```python
from build123d import *
from build123d.topology import SkipClean

# Parameters (mm, degrees)
SKETCH7_W       = 80
SKETCH7_H       = 28
EXTRUDE2_DEPTH  = 4
SKETCH8_W       = 28
SKETCH8_H       = 20
EXTRUDE3_DEPTH  = 9.5
EXTRUDE6_DEPTH  = 28
SKETCH15_R      = 7.5
EXTRUDE7_DEPTH  = 25
SKETCH16_W      = 3
SKETCH16_H      = 3
SKETCH8_4_W     = 28
SKETCH8_4_H     = 20
EXTRUDE8_DEPTH  = 9.5
EXTRUDE9_DEPTH  = 28
SKETCH19_R      = 7.5
EXTRUDE10_DEPTH = 25
SKETCH20_W      = 3
SKETCH20_H      = 3
FILLET1_R       = 2.5
EXTRUDE11_DEPTH = 16
SKETCH25_W      = 28
SKETCH25_H      = 5
EXTRUDE13_DEPTH = 12
EXTRUDE14_REACH = 90.69
FILLET11_R      = 2
SKETCH27_W      = 28
SKETCH27_H      = 5
EXTRUDE15_DEPTH = 12
EXTRUDE16_REACH = 90.69
FILLET14_R      = 2
SKETCH30_W      = 3
SKETCH30_H      = 3
EXTRUDE17_DEPTH = 12
SKETCH31_W      = 3
SKETCH31_H      = 3
EXTRUDE18_DEPTH = 12
SKETCH32_R      = 4
EXTRUDE19_DEPTH = 40
FILLET15_R      = 2
FILLET16_R      = 2
FILLET17_R      = 2
FILLET18_R      = 2
FILLET19_R      = 2
FILLET20_R      = 2
FILLET21_R      = 2
SKETCH33_R      = 1.5
EXTRUDE20_DEPTH = 59.523499692


with BuildPart() as part:
    # Sketch7 → Extrude2 (new body)
    with BuildSketch(Plane(origin=(0, 0, 0), x_dir=(1, 0, 0), z_dir=(0, 1, 0))):
        with Locations((0, 23)):
            Rectangle(SKETCH7_W, SKETCH7_H)
    extrude(amount=EXTRUDE2_DEPTH)


with BuildPart() as body_2:
    # Sketch8 → Extrude3 (new body)
    with BuildSketch(Plane(origin=(0, 4, 0), x_dir=(1, 0, 0), z_dir=(0, 1, 0))):
        with Locations((-23, 24)):
            Rectangle(SKETCH8_W, SKETCH8_H)
    extrude(amount=EXTRUDE3_DEPTH)

    # Sketch10 → Extrude6 (cut)
    with BuildSketch(Plane(origin=(-9, 0, 0), x_dir=(0, 0, -1), z_dir=(1, 0, 0))):
        with BuildLine():
            Line((31.5, 13.5), (24, 13.5))
            Line((24, 13.5), (16.5, 13.5))
            ThreePointArc((16.5, 13.5), (17.126403912, 10.499387259), (18.900980486, 8))
            Line((18.900980486, 8), (29.099019514, 8))
            ThreePointArc((29.099019514, 8), (30.873596088, 10.499387259), (31.5, 13.5))
        make_face()
    extrude(amount=-EXTRUDE6_DEPTH, mode=Mode.SUBTRACT)

    # Sketch15 → Extrude7 (cut)
    with SkipClean():  # the faces are left unmerged after this step: merging them gives an invalid solid
        with BuildSketch(Plane.ZY.offset(35.5)):
            with Locations((-24, 13.5)):
                Circle(SKETCH15_R)
        extrude(amount=-EXTRUDE7_DEPTH, mode=Mode.SUBTRACT)


with BuildPart() as cut_sweep1_tool:
    # Cut-Sweep1: sweep along a path in Sketch17
    with SkipClean():  # the faces are left unmerged after this step: merging them gives an invalid solid
        with BuildLine(Plane(origin=(-23, 0, 0), x_dir=(0, 0, -1), z_dir=(1, 0, 0))) as cut_sweep1_path:
            CenterArc((24, 13.5), 12.806248475, 0, 360)
        # Sketch16 → Cut-Sweep1 (sweep)
        with BuildSketch(Plane.XY.offset(-14)):
            with Locations((-23, 5.5)):
                Rectangle(SKETCH16_W, SKETCH16_H)
        sweep(path=cut_sweep1_path.line)


with BuildPart() as part_1:
    with SkipClean():  # the faces are left unmerged after this step: merging them gives an invalid solid
        add(part.part)

        # Cut-Sweep1: cut by cut_sweep1_tool
        add(cut_sweep1_tool.part, mode=Mode.SUBTRACT)

    # Sketch8<4> → Extrude8 (add)
    with BuildSketch(Plane(origin=(0, 4, 0), x_dir=(1, 0, 0), z_dir=(0, 1, 0))):
        with Locations((23, 24)):
            Rectangle(SKETCH8_4_W, SKETCH8_4_H)
    extrude(amount=EXTRUDE8_DEPTH)

    # Sketch18 → Extrude9 (cut)
    with BuildSketch(Plane(origin=(37, 0, 0), x_dir=(0, 0, -1), z_dir=(1, 0, 0))):
        with BuildLine():
            Line((18.900980486, 8), (29.099019514, 8))
            ThreePointArc((29.099019514, 8), (30.873596088, 10.499387259), (31.5, 13.5))
            Line((31.5, 13.5), (16.5, 13.5))
            ThreePointArc((16.5, 13.5), (17.126403912, 10.499387259), (18.900980486, 8))
        make_face()
    extrude(amount=-EXTRUDE9_DEPTH, mode=Mode.SUBTRACT)

    # Sketch19 → Extrude10 (cut)
    with BuildSketch(Plane(origin=(35.5, 0, 0), x_dir=(0, 0, -1), z_dir=(1, 0, 0))):
        with Locations((24, 13.5)):
            Circle(SKETCH19_R)
    extrude(amount=-EXTRUDE10_DEPTH, mode=Mode.SUBTRACT)

    # Cut-Sweep2: sweep along a path in Sketch21
    with BuildLine(Plane(origin=(23, 0, 0), x_dir=(0, 0, -1), z_dir=(1, 0, 0))) as cut_sweep2_path:
        CenterArc((24, 13.5), 12.806248475, 0, 360)
    # Sketch20 → Cut-Sweep2 (sweep, cut)
    with BuildSketch(Plane.XY.offset(-14)):
        with Locations((23, 5.5)):
            Rectangle(SKETCH20_W, SKETCH20_H)
    sweep(path=cut_sweep2_path.line, mode=Mode.SUBTRACT)

    # Fillet1
    fillet1_edges = [part_1.edges().sort_by_distance(p)[0] for p in [
        (-40, 2, -37),
        (40, 2, -37),
    ]]
    fillet(fillet1_edges, radius=FILLET1_R)

    # Sketch22 → Extrude11 (add)
    with BuildSketch(Plane(origin=(0, 0, 0), x_dir=(1, 0, 0), z_dir=(0, 1, 0))):
        Polygon((36.784969303, -11.093941854), (40, 9), (-40, 9), (-32, -41), (-16, -41), (-11.215030697, -11.093941854), align=None)
        Polygon((12.66820222, 4), (11.053171523, -6.093941854), (-5.351435136, -6.093941854), (-3.73640444, 4), align=None, mode=Mode.SUBTRACT)
        Polygon((17.73179778, 4), (34.13640444, 4), (32.521373743, -6.093941854), (16.116767084, -6.093941854), align=None, mode=Mode.SUBTRACT)
    extrude(amount=EXTRUDE11_DEPTH)



with BuildPart() as body_2_1:
    with SkipClean():  # the faces are left unmerged after this step: merging them gives an invalid solid
        add(body_2.part)

        # Cut-Sweep1: cut by cut_sweep1_tool
        add(cut_sweep1_tool.part, mode=Mode.SUBTRACT)


with BuildPart() as part_2:
    with SkipClean():  # the faces are left unmerged after this step: merging them gives an invalid solid
        add(part_1.part)

        add(body_2_1.part)  # Extrude13 merges body 2
        # Sketch25 → Extrude13 (add)
        with BuildSketch(Plane(origin=(0, 4, 0), x_dir=(-1, 0, 0), z_dir=(0, 1, 0))):
            with Locations((23, -11.5)):
                Rectangle(SKETCH25_W, SKETCH25_H)
        extrude(amount=EXTRUDE13_DEPTH)

    # Sketch26 → Extrude14 (cut, up to next)
    with BuildSketch(Plane.ZY.offset(37), mode=Mode.PRIVATE) as extrude14_sk1:
        Polygon((-14, 13.5), (-9, 16), (-14, 16), align=None)
    extrude14_tool1 = extrude(extrude14_sk1.sketch, amount=-EXTRUDE14_REACH, mode=Mode.PRIVATE) & part_2.part
    add(extrude14_tool1.solids().sort_by_distance((-37, 15.166667, -12.333333))[0], mode=Mode.SUBTRACT)

    # Fillet11
    fillet11_edges = [part_2.edges().sort_by_distance(p)[0] for p in [
        (-9, 10, -9),
    ]]
    fillet(fillet11_edges, radius=FILLET11_R)

    # Sketch27 → Extrude15 (add)
    with SkipClean():  # the faces are left unmerged after this step: merging them gives an invalid solid
        with BuildSketch(Plane(origin=(0, 4, 0), x_dir=(-1, 0, 0), z_dir=(0, 1, 0))):
            with Locations((-23, -11.5)):
                Rectangle(SKETCH27_W, SKETCH27_H)
        extrude(amount=EXTRUDE15_DEPTH)

    # Sketch28 → Extrude16 (cut, up to next)
    with BuildSketch(Plane(origin=(37, 0, 0), x_dir=(0, 0, -1), z_dir=(1, 0, 0)), mode=Mode.PRIVATE) as extrude16_sk1:
        Polygon((14, 13.5), (9, 16), (14, 16), align=None)
    extrude16_tool1 = extrude(extrude16_sk1.sketch, amount=-EXTRUDE16_REACH, mode=Mode.PRIVATE) & part_2.part
    add(extrude16_tool1.solids().sort_by_distance((37, 15.166667, -12.333333))[0], mode=Mode.SUBTRACT)

    # Fillet14
    fillet14_edges = [part_2.edges().sort_by_distance(p)[0] for p in [
        (9, 10, -9),
    ]]
    fillet(fillet14_edges, radius=FILLET14_R)

    # Sketch30 → Extrude17 (cut)
    with SkipClean():  # the faces are left unmerged after this step: merging them gives an invalid solid
        with BuildSketch(Plane(origin=(0, 16, 0), x_dir=(-1, 0, 0), z_dir=(0, 1, 0))):
            with Locations((-23, -12.5)):
                Rectangle(SKETCH30_W, SKETCH30_H)
        extrude(amount=-EXTRUDE17_DEPTH, mode=Mode.SUBTRACT)

    # Sketch31 → Extrude18 (cut)
    with SkipClean():  # the faces are left unmerged after this step: merging them gives an invalid solid
        with BuildSketch(Plane(origin=(0, 16, 0), x_dir=(-1, 0, 0), z_dir=(0, 1, 0))):
            with Locations((23, -12.5)):
                Rectangle(SKETCH31_W, SKETCH31_H)
        extrude(amount=-EXTRUDE18_DEPTH, mode=Mode.SUBTRACT)

    # Sketch32 → Extrude19 (cut)
    with SkipClean():  # the faces are left unmerged after this step: merging them gives an invalid solid
        with BuildSketch(Plane.XY.offset(41)):
            with Locations((-24, 8)):
                Circle(SKETCH32_R)
        extrude(amount=-EXTRUDE19_DEPTH, mode=Mode.SUBTRACT)

    # Fillet15
    fillet15_edges = [part_2.edges().sort_by_distance(p)[0] for p in [
        (-40, 10, -9),
    ]]
    fillet(fillet15_edges, radius=FILLET15_R)

    # Fillet16
    # the kernel refuses this fillet: 2 mm, written as the material it adds along each edge
    with BuildSketch(Plane(origin=(-37, -0.417336402, -9), x_dir=(0, 0, -1), z_dir=(0, 1, 0))) as fillet16_piece_1_section:
        with BuildLine():
            CenterArc((1.766934561, 2), FILLET16_R, 199.655233066, 70.344766934)
            Line((-0.11653272, 1.327280888), (-0.304879448, 1.260008977))
            ThreePointArc((-0.304879448, 1.260008977), (-0.2, 0.654561776), (-0.2, 0))
            Line((-0.2, 0), (0, -0.2))
            Line((0, -0.2), (1.766934561, -0.2))
            Line((1.766934561, -0.2), (1.766934561, 0))
        make_face()
    fillet16_piece_1 = extrude(amount=16.417336402, mode=Mode.PRIVATE)
    fillet16_piece_1 = split(fillet16_piece_1, bisect_by=Plane(origin=(-37.361885023, 0, -9.612553635), z_dir=(0, 1, 0)), keep=Keep.TOP, mode=Mode.PRIVATE)
    fillet16_piece_1 = split(fillet16_piece_1, bisect_by=Plane(origin=(-37.361885023, 14.554978546, -11.890042908), z_dir=(0, -0.8944271909999159, 0.44721359549995804)), keep=Keep.TOP, mode=Mode.PRIVATE)
    add(fillet16_piece_1)

    # Fillet17
    fillet17_edges = [part_2.edges().sort_by_distance(p)[0] for p in [
        (40, 10, -9),
    ]]
    fillet(fillet17_edges, radius=FILLET17_R)

    # Fillet18
    # the kernel refuses this fillet: 2 mm, written as the material it adds along each edge
    with BuildSketch(Plane(origin=(37, -0.417336402, -9), x_dir=(0.9961678888786428, 0, 0.08746163254289245), z_dir=(0, 1, 0))) as fillet18_piece_1_section:
        with BuildLine():
            CenterArc((1.837796796, 1.935086736), FILLET18_R, 185.017593378, 70.344766934)
            Line((-0.154538981, 1.760163471), (-0.353772559, 1.742671145))
            Line((-0.353772559, 1.742671145), (-0.199233578, -0.017492327))
            Line((-0.199233578, -0.017492327), (0.017492327, -0.199233578))
            ThreePointArc((0.017492327, -0.199233578), (0.669545749, -0.141984536), (1.281845737, -0.193508674))
            Line((1.281845737, -0.193508674), (1.332386742, 0))
        make_face()
    fillet18_piece_1 = extrude(amount=16.417336402, mode=Mode.PRIVATE)
    fillet18_piece_1 = split(fillet18_piece_1, bisect_by=Plane(origin=(37.361885023, 14.554978546, -11.890042908), z_dir=(0, -0.8944271909999157, 0.4472135954999582)), keep=Keep.TOP, mode=Mode.PRIVATE)
    fillet18_piece_1 = split(fillet18_piece_1, bisect_by=Plane(origin=(37.361885023, 0, -9.612553635), z_dir=(0, 1, 0)), keep=Keep.TOP, mode=Mode.PRIVATE)
    add(fillet18_piece_1)

    # Fillet19
    fillet19_edges = [part_2.edges().sort_by_distance(p)[0] for p in [
        (11.053171523, 8, 6.093941854),
        (32.521373743, 8, 6.093941854),
    ]]
    fillet(fillet19_edges, radius=FILLET19_R)

    # Fillet20
    fillet20_edges = [part_2.edges().sort_by_distance(p)[0] for p in [
        (36.784969303, 8, 11.093941854),
        (-3.73640444, 8, -4),
        (-5.351435136, 8, 6.093941854),
        (12.66820222, 8, -4),
        (34.13640444, 8, -4),
        (17.73179778, 8, -4),
        (16.116767084, 8, 6.093941854),
    ]]
    fillet(fillet20_edges, radius=FILLET20_R)

    # Fillet21
    fillet21_edges = [part_2.edges().sort_by_distance(p)[0] for p in [
        (-11.215030697, 8, 11.093941854),
    ]]
    fillet(fillet21_edges, radius=FILLET21_R)

    # Sketch33 → Extrude20 (cut, through all)
    with BuildSketch(Plane(origin=(0, 4, 0), x_dir=(-1, 0, 0), z_dir=(0, 1, 0))):
        with Locations(Location((0, -13.5, 0), (0, 0, 90))):
            Circle(SKETCH33_R)
        with Locations(Location((0, -22, 0), (0, 0, 90))):
            Circle(SKETCH33_R)
    extrude(amount=-EXTRUDE20_DEPTH, mode=Mode.SUBTRACT)


solid = part_2.part
```
Build history of the part. All positions in model axes, mm. A direction names the side the tool comes from. Give positions to 0.01 mm unless a question says otherwise; leave off trailing zeros. Loops run counter-clockwise (first coordinate to the right, second up) from the corner with the lowest first, then second, coordinate; pieces in that order, holes last.
Item 1: Which spindle directions (+Z, -Z, +X, -X, +Y, -Y) get a long thin tool onto all of the face, cutting with end or side? Do faces 3 (the face through (16.956, 8.112, 5.41)), 4 (the face through (22.7, 15.3, -10.4)), 5 (the face through (-35.5, 7, -24)), 6 (the face through (-27.2, 5.6, 21.3)), 7 (the face through (21.5, 3, -18)). Say none if no direction does.
Answers follow:
face 3: +Y, -Y
face 4: -Z, +X, -X, +Y
face 5: +Y
face 6: +Z
face 7: none
Item 2: Slice it at C-C, the plane z = 33. List the corners of the cut face in (x, y).
Answers follow:
outline: (-33.28, 0) - (-14.72, 0) - (-14.72, 16) - (-33.28, 16) - close; hole circle Ø8 at (-24, 8)
Item 3: Slice it at A-A, the plane x = 28. List the corners of the cut face in (y, z).
Answers follow:
outline: (0, -37) - (4, -37) - (4, -34) - (13.5, -34) - (13.5, -31.5) arc R7.5 cw to (13.5, -16.5) - (13.5, -14) - (16, -9) - (16, -4) - (0, -4) - close; (0, 6.09) - (16, 6.09) - (16, 11.09) - (0, 11.09) - close
Item 4: Pull direction X, two halves, no side cores. Call faces 1 (the face through (33.33, 8.11, -3.28)), 2 (the face through (-23, 13.5, -33)): released by +X, released by -X, zero draft, split by the parting line, or undercut.
Answers follow:
face 1: undercut
face 2: zero draft
Item 5: Slice it at B-B, the plane x = 0. List the corners of the cut face in (y, z), and give its area (3 significant figures).
Answers follow:
outline: (0, -37) - (4, -37) - (4, -23.5) - (0, -23.5) - close; (0, -20.5) - (4, -20.5) - (4, -15) - (0, -15) - close; (0, -12) - (4, -12) - (4, -9) - (16, -9) - (16, -4) - (0, -4) - close; (0, 6.09) - (16, 6.09) - (16, 11.09) - (0, 11.09) - close
area: 248 mm2
Item 6: Flat gauge pins, fed straight in: pin 1 (8 mm diameter, centred on x = 2, y = 7, fed in from +Z); pin 2 (0.6 mm diameter, centred on y = 7, z = -23, fed in from +X); pin 3 (1.5 mm diameter, centred on x = -6.5, y = 5.5, fed in from -Z); pin 4 (9 mm diameter, centred on x = -22, y = 7.5, fed in from +Z). Where does each tip first touch, or does it go through?
Answers follow:
pin 1: stops at z = 11.09
pin 2: stops at x = 37
pin 3: stops at z = -9.02
pin 4: stops at z = 41
Item 7: Drill centre lines: line 1 (Z direction, x = 20, y = 6.75); line 2 (Z direction, x = 4, y = 13); line 3 (X direction, y = 2.35, z = -22). Where is each one in solid material? Low to high.
Answers follow:
line 1: z = -34 to -27.27, -20.73 to -4, 6.09 to 11.09
line 2: z = -9 to -4, 6.09 to 11.09
line 3: x = -40 to -1.5, 1.5 to 40
